Check sheet for the modelled part. Datum: model origin and axes. Units: mm. Face numbers are marked on the shaded views. A direction names the side the tool comes from. Round coordinates to 2 decimals unless told otherwise and drop trailing zeros. Order: outer loops, then holes, each group sorted by start corner. A loop starts at its lowest first (then second) coordinate and runs counter-clockwise, first axis right, second up.
(1) Tool access check on the marked faces 1 and 2. Record the directions out of +Z, -Z, +X, -X, +Y, -Y that give a thin tool (end or side, any length) a straight path to the whole face; none if there is none.
(2) Sectioned sample at C-C, the plane z = 12. Enter the section's corners in (x, y).
(3) Thickness scan on probe 1 along Y at (x, z) = (0, 5.8); probe 2 along Z at (x, y) = (-6.25, 7.25); probe 3 along Y at (x, z) = (-2, 2.5). Record the ranges inside material, lowest first.
(4) Sectioned sample at D-D, the plane x = -4. Enter the section's corners in (y, z), and give its area (3 significant figures).
(5) Mould release check, pull along Y, two halves, no side actions. Record for the marked faces 3, 4 and 5: released by +Y, released by -Y, zero draft, split by the parting line, or undercut.
(6) Sectioned sample at A-A, the plane y = 0. Enter the section's corners in (x, z), and give its area (3 significant figures).
(7) Depth check by flat-ended pin: pin 1 (4 mm diameter, centred on x = 1.5, y = -3.5, fed in from -Z); pin 2 (8 mm diameter, centred on x = 5, z = 4, fed in from -Y); pin 3 (5 mm diameter, centred on x = 8, z = 24, fed in from -Y); pin 4 (1.5 mm diameter, centred on x = 0.5, y = 0, fed in from -Z). Enter the tip coordinate at first touch or a pass-through.
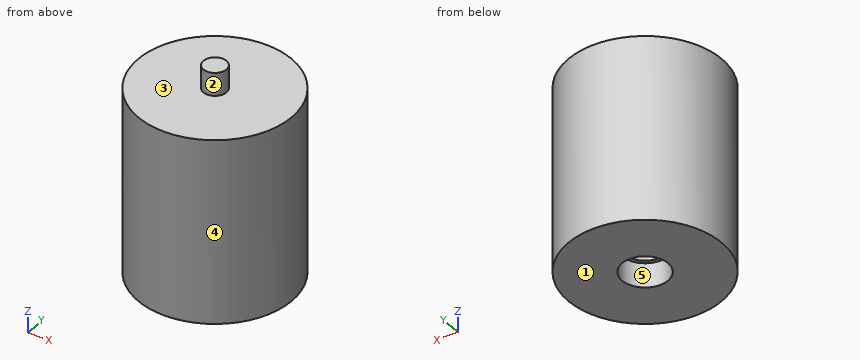
```python
from build123d import *

# Parameters (mm, degrees)
SKETCH_R        = 10
PAD_DEPTH       = 24
SKETCH001_R     = 1.5
PAD001_DEPTH    = 3
SKETCH002_R     = 3
POCKET_DEPTH    = 3.16
SKETCH003_R     = 2.5
POCKET001_DEPTH = 3.4


with BuildPart() as part:
    # Sketch → Pad (new body)
    with BuildSketch(Plane.XY):
        Circle(SKETCH_R)
    extrude(amount=PAD_DEPTH)

    # Sketch001 → Pad001 (new body)
    with BuildSketch(Plane.XY.offset(24)):
        Circle(SKETCH001_R)
    extrude(amount=PAD001_DEPTH)

    # Sketch002 → Pocket (cut)
    with BuildSketch(Plane(origin=(0, 0, 0), x_dir=(1, 0, 0), z_dir=(0, 0, -1))):
        Circle(SKETCH002_R)
    extrude(amount=-POCKET_DEPTH, mode=Mode.SUBTRACT)

    # Sketch003 → Pocket001 (cut)
    with BuildSketch(Plane(origin=(0, 0, 3.16), x_dir=(1, 0, 0), z_dir=(0, 0, -1))):
        Circle(SKETCH003_R)
    extrude(amount=-POCKET001_DEPTH, mode=Mode.SUBTRACT)


solid = part.part
```
Derived:
1. face 1: -Z, +X, -X, +Y, -Y
1. face 2: +Z
2. outline: circle Ø20 at (0, 0)
3. probe 1: y = -10 to -2.5, 2.5 to 10
3. probe 2: z = 0 to 24
3. probe 3: y = -9.8 to -2.24, 2.24 to 9.8
4. outline: (-9.17, 0) - (9.17, 0) - (9.17, 24) - (-9.17, 24) - close
4. area: 440 mm2
5. face 3: zero draft
5. face 4: split by the parting line
5. face 5: undercut
6. outline: (-10, 0) - (-3, 0) - (-3, 3.16) - (-2.5, 3.16) - (-2.5, 6.56) - (2.5, 6.56) - (2.5, 3.16) - (3, 3.16) - (3, 0) - (10, 0) - (10, 24) - (1.5, 24) - (1.5, 27) - (-1.5, 27) - (-1.5, 24) - (-10, 24) - close
6. area: 453 mm2
7. pin 1: stops at z = 0
7. pin 2: stops at y = -9.95
7. pin 3: stops at y = -8.35
7. pin 4: stops at z = 6.56
